Autodesk Inventor part; units mm, degrees
ref_plane "YZ Plane" through (0, 0, 0) normal (1, 0, 0) x (0, 1, 0)
ref_plane "XZ Plane" through (0, 0, 0) normal (0, 1, 0) x (-1, 0, 0)
ref_plane "XY Plane" through (0, 0, 0) normal (0, 0, 1) x (1, 0, 0)
sketch "스케치1" plane through (0, 0, 0) normal (0, 0, 1) x (1, 0, 0)
  line L0 (-100, 100) -> (100, 100)
  line L1 (100, 100) -> (100, -100)
  line L2 (100, -100) -> (-100, -100)
  line L3 (-100, -100) -> (-100, 100)
  point P0 (0, 0)
  dimension "d0" = 200
  dimension "d1" = 200
  dimension "d2" = 100
  dimension "d3" = 100
extrude "돌출1" add sketch "스케치1" along normal blind 150
sketch "스케치2" plane through (0, 0, 150) normal (0, 0, 1) x (1, 0, 0)
  line L0 (-90, 90) -> (90, 90)
  line L1 (90, 90) -> (90, -90)
  line L2 (90, -90) -> (-90, -90)
  line L3 (-90, -90) -> (-90, 90)
  point P0 (0, 0)
  dimension "d6" = 180
  dimension "d7" = 180
  dimension "d8" = 90
  dimension "d9" = 90
extrude "돌출2" cut sketch "스케치2" against normal blind 140
properties part number "basket"
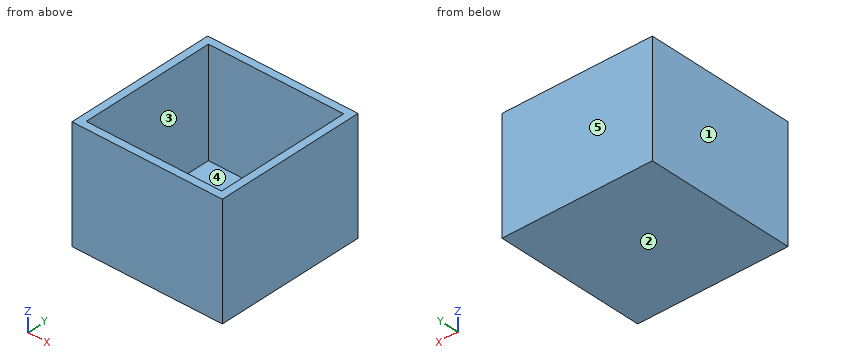
Part model, mm, in its own coordinate system. Face numbers are marked on the shaded views. A direction names the side the tool comes from. Round coordinates to 2 decimals unless told otherwise and drop trailing zeros. Write each loop counter-clockwise with the first axis right and the second up, starting at its lowest first coordinate (ties: lowest second). Pieces come first, ordered by that corner, then holes. Notation, with made-up numbers: M 88.5,-30 L 102.5,-30 A32 cw 102.5,-3 Z; hole C 29.5,-23.75 d7. An arc over 180 degrees is marked long. Answer as CSV lines item,"result". Start each with the question number.
1) Which spindle directions (+Z, -Z, +X, -X, +Y, -Y) get a long thin tool onto all of the face, cutting with end or side? Do the marked faces 4 and 5. Say none if no direction does.
2) Drop a flat-ended pin along its axis: pin 1 (12 mm diameter, centred on x = -44, y = -67.5, fed in from +Z). Give the stop position or say it passes through.
3) Band-saw the part on B-B (x = -47). List the corners of the cut face in (y, z), then the cut area to 3 significant figures.
4) Mould opens along X. For the marked faces 1, 2 and 3 say: +X half, -X half, draft (parallel to the pull), parting line (faces both ways), or undercut.
5) Band-saw the part on A-A (z = 75.5). List the corners of the cut face in (x, y), then the cut area to 3 significant figures.
6) Drill centre lines: L1, parallel to Y at x = 26.5, z = 48; L2, parallel to Z at x = -11.5, y = -74. Where is each one in solid material? Low to high.
Worked out:
1,face 4,"+Z"
1,face 5,"+Z, -Z, +X, -X, +Y"
2,pin 1,"z = 10"
3,outline,"M -100,0 L 100,0 L 100,150 L 90,150 L 90,10 L -90,10 L -90,150 L -100,150 Z"
3,area,"4,800 mm²"
4,face 1,"-X half"
4,face 2,"draft"
4,face 3,"undercut"
5,outline,"M -100,-100 L 100,-100 L 100,100 L -100,100 Z; hole M -90,-90 L 90,-90 L 90,90 L -90,90 Z"
5,area,"7,600 mm²"
6,L1,"-100 to -90, 90 to 100"
6,L2,"0 to 10"
